from build123d import *

# Parameters (mm, degrees)
CONG_1_R = 0.25


with BuildPart() as part:
    # Esquisse1 → Révolution1 (revolve)
    with BuildSketch(Plane.XY, mode=Mode.PRIVATE) as r_volution1_sk:
        Polygon((4, 5), (4, 0), (9, 0), (9, 1), (8, 1), (8, 5), align=None)
    revolve(r_volution1_sk.sketch.rotate(Axis((0, 0, 0), (0, 1, 0)), 90), axis=Axis((0, 0, 0), (0, 1, 0)))

    # Congé1
    cong_1_edges = [part.edges().sort_by_distance(p)[0] for p in [
        (0, 5, 8),
        (0, 0, 9),
        (0, 0, 4),
        (0, 5, 4),
    ]]
    fillet(cong_1_edges, radius=CONG_1_R)


solid = part.part
Can you work these out from the model? Positions are in its coordinate system, mm. A direction names the side the tool comes from. Give positions to 0.01 mm unless a question says otherwise; leave off trailing zeros. Write each loop counter-clockwise with the first axis right and the second up, starting at its lowest first coordinate (ties: lowest second). Pieces come first, ordered by that corner, then holes. Notation, with made-up numbers: (16, -34) -> (62, -34) arc R19 ccw to (62, -4) -> close; hole circle Ø5 at (48, -25). An arc over 180 degrees is marked (long way). Answer as a JSON object with one key per item and string values. Group by question number.
Item 1: Suppose I cut it at C-C (y = 4.2). Please give me the cut outline in (x, z), plus the area to 3 significant figures.
Item 2: Please list where these lines run through material, in increasing order: line 1 (X direction, y = 2.1, z = 0); line 2 (X direction, y = 1.25, z = 2.25); line 3 (Y direction, x = 7.25, z = 3.5). Write a range as [from, to].
Item 3: For faces 4 (the face through (7.81, 2.9, 1.73)), 5 (the face through (3.3, 5, -3.3)), which set-ups out of +Z, -Z, +X, -X, +Y, -Y let a thin tool reach every point of the face, with its end or its side?
Item 4: I'm going to push flat-ended pins straight in: P1, Ø1, axis at x = -1, z = -3.5, coming from the +Y side; P2, Ø3, axis at x = 0.5, z = 0, coming from the +Y side. Where does each tip first touch, or does it pass through?
Item 5: We'd pull the mould along Z, two halves only. Please class faces 1 (the face through (4, 0, -2)), 2 (the face through (3.905, 2.468, 0.867)), 3 (the face through (-6.083, 0.63, 6.633)): +Z half, -Z half, draft (parallel to the pull), parting line (faces both ways), or undercut.
Item 6: Suppose I cut it at B-B (x = 0). Please give me the cut outline in (y, z), plus the area to 3 significant figures.
Item 7: Suppose I cut it at A-A (z = 0). Please give me the cut outline in (x, y).
Findings:
{
 "1": {"outline": "circle Ø16 at (0, 0); hole circle Ø8 at (0, 0)", "area": "151 mm²"},
 "2": {"line 1": "x = [-8, -4], [4, 8]", "line 2": "x = [-7.68, -3.31], [3.31, 7.68]", "line 3": "y = [0, 1]"},
 "3": {"face 4": "+Y", "face 5": "+Z, -Z, +X, -X, +Y"},
 "4": {"P1": "stops at y = 4.97", "P2": "passes through"},
 "5": {"face 1": "draft", "face 2": "undercut", "face 3": "parting line"},
 "6": {"outline": "(0, -8.75) arc R0.25 ccw to (0.25, -9) -> (1, -9) -> (1, -8) -> (4.75, -8) arc R0.25 ccw to (5, -7.75) -> (5, -4.25) arc R0.25 ccw to (4.75, -4) -> (0.25, -4) arc R0.25 ccw to (0, -4.25) -> close; (0, 4.25) arc R0.25 ccw to (0.25, 4) -> (4.75, 4) arc R0.25 ccw to (5, 4.25) -> (5, 7.75) arc R0.25 ccw to (4.75, 8) -> (1, 8) -> (1, 9) -> (0.25, 9) arc R0.25 ccw to (0, 8.75) -> close", "area": "41.9 mm²"},
 "7": {"outline": "(-9, 0.25) arc R0.25 ccw to (-8.75, 0) -> (-4.25, 0) arc R0.25 ccw to (-4, 0.25) -> (-4, 4.75) arc R0.25 ccw to (-4.25, 5) -> (-7.75, 5) arc R0.25 ccw to (-8, 4.75) -> (-8, 1) -> (-9, 1) -> close; (4, 0.25) arc R0.25 ccw to (4.25, 0) -> (8.75, 0) arc R0.25 ccw to (9, 0.25) -> (9, 1) -> (8, 1) -> (8, 4.75) arc R0.25 ccw to (7.75, 5) -> (4.25, 5) arc R0.25 ccw to (4, 4.75) -> close"}
}
